The listing builds one solid part. Answer for the finished solid, in the listing's coordinates (mm). Coordinates: 2 decimals unless noted, no trailing zeros. Write each loop counter-clockwise with the first axis right and the second up, starting at its lowest first coordinate (ties: lowest second). Pieces come first, ordered by that corner, then holes.
from build123d import *

# Parameters (mm, degrees)
F1_DEPTH = 4.5


with BuildPart() as f1:
    # F0 (on Top) → F1 (new body)
    with BuildSketch(Plane.XY):
        with BuildLine():
            Line((86.379995, 144.308884), (-90.620005, 144.308884))
            ThreePointArc((-90.620005, 144.308884), (-100.5195, 140.208379), (-104.620005, 130.308884))
            Line((-104.620005, 130.308884), (-104.620005, -123.691116))
            ThreePointArc((-104.620005, -123.691116), (-100.5195, -133.590611), (-90.620005, -137.691116))
            Line((-90.620005, -137.691116), (86.379995, -137.691116))
            ThreePointArc((86.379995, -137.691116), (96.27949, -133.590611), (100.379995, -123.691116))
            Line((100.379995, -123.691116), (100.379995, 130.308884))
            ThreePointArc((100.379995, 130.308884), (96.27949, 140.208379), (86.379995, 144.308884))
        make_face()
        with BuildLine():
            ThreePointArc((-65.620005, 117.308884), (-61.812393, 126.501272), (-52.620005, 130.308884))
            Line((-52.620005, 130.308884), (48.379995, 130.308884))
            ThreePointArc((48.379995, 130.308884), (57.572383, 126.501272), (61.379995, 117.308884))
            ThreePointArc((61.379995, 117.308884), (57.572383, 108.116496), (48.379995, 104.308884))
            Line((48.379995, 104.308884), (-52.620005, 104.308884))
            ThreePointArc((-52.620005, 104.308884), (-61.812393, 108.116496), (-65.620005, 117.308884))
        make_face(mode=Mode.SUBTRACT)
    extrude(amount=F1_DEPTH)


solid = f1.part
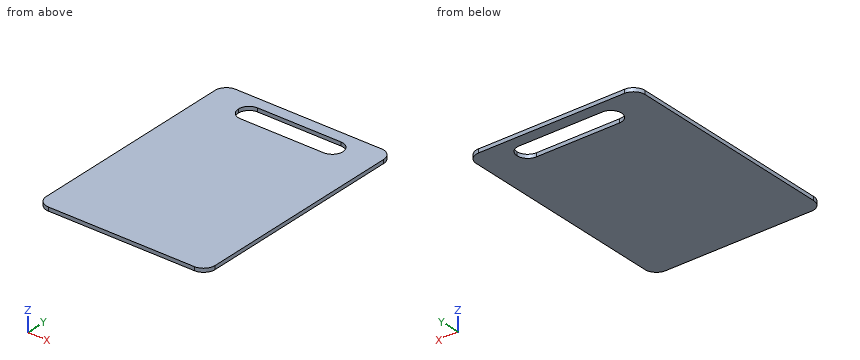
Q1. The part is cut by section A-A, the plane x = -42.5. Write down the section's boundary in (y, z), then the cut area to 3 significant figures.
Answers below:
outline: (-137.69, 0) - (104.31, 0) - (104.31, 4.5) - (-137.69, 4.5) - close; (130.31, 0) - (144.31, 0) - (144.31, 4.5) - (130.31, 4.5) - close
area: 1,150 mm2
Q2. The part is cut by section B-B, the plane z = 2.8. Write down the section's boundary in (x, y), then the cut area to 3 significant figures.
Answers below:
outline: (-104.62, -123.69) arc R14 ccw to (-90.62, -137.69) - (86.38, -137.69) arc R14 ccw to (100.38, -123.69) - (100.38, 130.31) arc R14 ccw to (86.38, 144.31) - (-90.62, 144.31) arc R14 ccw to (-104.62, 130.31) - close; hole (-65.62, 117.31) arc R13 ccw to (-52.62, 104.31) - (48.38, 104.31) arc R13 ccw to (61.38, 117.31) arc R13 ccw to (48.38, 130.31) - (-52.62, 130.31) arc R13 ccw to start
area: 54,500 mm2
Q3. Find the intervals of material crossed by probe 1 along X at (y, z) = (117.5, 0.9); probe 2 along Y at (x, z) = (-47, 3.6); probe 3 along X at (y, z) = (123, 1), in increasing order.
Answers below:
probe 1: x = -104.62 to -65.62, 61.38 to 100.38
probe 2: y = -137.69 to 104.31, 130.31 to 144.31
probe 3: x = -104.62 to -64.31, 60.07 to 100.38
